from build123d import *

# Parameters (mm, degrees)
F0_R     = 1.35
F0_W     = 33.5
F0_H     = 25
F1_DEPTH = 15
F0_R_2   = 0.75
F0_W_2   = 24.5
F0_H_2   = 24.5
F2_DEPTH = 3
F3_DEPTH = 8
F4_DEPTH = 4


with BuildPart() as f1:
    # F0 (on Top) → F1 (new body)
    with BuildSketch(Plane.XY):
        with BuildLine():
            ThreePointArc((-20.740295, 15.731344), (-23.568722, 14.559771), (-24.740295, 11.731344))
            Line((-24.740295, 11.731344), (-24.740295, -20.268656))
            ThreePointArc((-24.740295, -20.268656), (-23.568722, -23.097083), (-20.740295, -24.268656))
            Line((-20.740295, -24.268656), (16.259705, -24.268656))
            ThreePointArc((16.259705, -24.268656), (19.088132, -23.097083), (20.259705, -20.268656))
            Line((20.259705, -20.268656), (20.259705, 11.731344))
            ThreePointArc((20.259705, 11.731344), (19.088132, 14.559771), (16.259705, 15.731344))
            Line((16.259705, 15.731344), (-20.740295, 15.731344))
        make_face()
        with Locations((-20.740295, -20.268656)):
            Circle(F0_R, mode=Mode.SUBTRACT)
        with Locations((16.259705, -20.268656)):
            Circle(F0_R, mode=Mode.SUBTRACT)
        with Locations((-20.740295, 11.731344)):
            Circle(F0_R, mode=Mode.SUBTRACT)
        with Locations((-2.240295, -4.268656)):
            Rectangle(F0_W, F0_H, mode=Mode.SUBTRACT)
        with Locations((16.259705, 11.731344)):
            Circle(F0_R, mode=Mode.SUBTRACT)
    extrude(amount=F1_DEPTH)

    # F0 (on Top) → F2 (join)
    with BuildSketch(Plane.XY):
        with Locations((-2.240295, -4.268656)):
            Rectangle(F0_W, F0_H)
        with Locations((-16.674155, -4.268656)):
            Circle(F0_R_2, mode=Mode.SUBTRACT)
        with Locations((-2.240295, -4.268656)):
            Rectangle(F0_W_2, F0_H_2, mode=Mode.SUBTRACT)
        with Locations((12.193565, -4.268656)):
            Circle(F0_R_2, mode=Mode.SUBTRACT)
    extrude(amount=F2_DEPTH)

    # F0 (on Top) → F3 (join)
    with BuildSketch(Plane.XY):
        with Locations((-16.674155, -4.268656)):
            Circle(F0_R_2)
        with Locations((12.193565, -4.268656)):
            Circle(F0_R_2)
    extrude(amount=F3_DEPTH)

    # F0 (on Top) → F4 (join)
    with BuildSketch(Plane.XY):
        with Locations((-20.740295, 11.731344)):
            Circle(F0_R)
        with Locations((16.259705, 11.731344)):
            Circle(F0_R)
        with Locations((16.259705, -20.268656)):
            Circle(F0_R)
        with Locations((-20.740295, -20.268656)):
            Circle(F0_R)
    extrude(amount=F4_DEPTH)


solid = f1.part
For this review, take the finished solid that the model builds, in its own axes (mm). A direction names the side the tool comes from. Round coordinates to 2 decimals unless told otherwise and drop trailing zeros. Loops run counter-clockwise (first coordinate to the right, second up) from the corner with the lowest first, then second, coordinate; pieces in that order, holes last. Notation, with made-up numbers: (67, 52) - (125, 52) arc R26 cw to (125, 85) - close; hole circle Ø11 at (-9.75, -26). An arc over 180 degrees is marked (long way). One line per question, with ' | ' between items.
Q1. Take a section at A-A (x = -12). Give the boundary of the cut face in (y, z), and give its area (4 significant figures).
Taken from the geometry:
outline: (-24.27, 0) - (-16.52, 0) - (-16.52, 3) - (-16.77, 3) - (-16.77, 15) - (-24.27, 15) - close; (7.98, 0) - (15.73, 0) - (15.73, 15) - (8.23, 15) - (8.23, 3) - (7.98, 3) - close | area: 226.5 mm²
Q2. Take a section at B-B (z = 11). Give the boundary of the cut face in (x, y).
Taken from the geometry:
outline: (-24.74, -20.27) arc R4 ccw to (-20.74, -24.27) - (16.26, -24.27) arc R4 ccw to (20.26, -20.27) - (20.26, 11.73) arc R4 ccw to (16.26, 15.73) - (-20.74, 15.73) arc R4 ccw to (-24.74, 11.73) - close; hole circle Ø2.7 at (-20.74, -20.27); hole circle Ø2.7 at (-20.74, 11.73); hole (-18.99, -16.77) - (14.51, -16.77) - (14.51, 8.23) - (-18.99, 8.23) - close; hole circle Ø2.7 at (16.26, -20.27); hole circle Ø2.7 at (16.26, 11.73)
Q3. For line 1 along X through (y, z) = (-10.5, 1.5); line 2 along X through (y, z) = (-5, 13.5); line 3 along Y through (x, z) = (-3.5, 6), list the stretches that pass through material, from the lowest coordinate up. Write a range as [from, to].
Taken from the geometry:
line 1: x = [-24.74, -14.49], [10.01, 20.26] | line 2: x = [-24.74, -18.99], [14.51, 20.26] | line 3: y = [-24.27, -16.77], [8.23, 15.73]
Q4. For pin 1 (1.5 mm diameter, centred on x = -18, y = 10, fed in from -Z); pin 2 (0.8 mm diameter, centred on x = 16, y = 12, fed in from +Z), all flat-tipped, find the tip position at first contact; note any pin that passes through.
Taken from the geometry:
pin 1: stops at z = 0 | pin 2: stops at z = 4
Q5. Take a section at D-D (z = 5). Give the boundary of the cut face in (x, y).
Taken from the geometry:
outline: (-24.74, -20.27) arc R4 ccw to (-20.74, -24.27) - (16.26, -24.27) arc R4 ccw to (20.26, -20.27) - (20.26, 11.73) arc R4 ccw to (16.26, 15.73) - (-20.74, 15.73) arc R4 ccw to (-24.74, 11.73) - close; circle Ø1.5 at (-16.67, -4.27); circle Ø1.5 at (12.19, -4.27); hole circle Ø2.7 at (-20.74, -20.27); hole circle Ø2.7 at (-20.74, 11.73); hole (-18.99, -16.77) - (14.51, -16.77) - (14.51, 8.23) - (-18.99, 8.23) - close; hole circle Ø2.7 at (16.26, -20.27); hole circle Ø2.7 at (16.26, 11.73)
Q6. Tool access review of faces 1 (the flat face through (-2, 7.981, 1)), 2 (the cylindrical face through (-23.54, 14.59, 7.4)), 3 (the flat face through (-18.99, -4, 9)): name each direction out of +Z, -Z, +X, -X, +Y, -Y from which nothing blocks a thin tool from reaching the whole face with its end or side.
Taken from the geometry:
face 1: +Z, -Z | face 2: +Z, -Z, -X, +Y | face 3: +Z
Q7. The part is to be moulded in two halves that separate along Y. For faces 4 (the flat face through (-15, -4, 3)), 5 (the cylindrical face through (19.12, 14.53, 7.4)), 6 (the flat face through (-3, 9, 15)), say which applies: released by +Y, released by -Y, zero draft, split by the parting line, or undercut.
Taken from the geometry:
face 4: undercut | face 5: released by +Y | face 6: zero draft
Q8. Take a section at C-C (y = -14.5). Give the boundary of the cut face in (x, z), and give its area (4 significant figures).
Taken from the geometry:
outline: (-24.74, 0) - (-14.49, 0) - (-14.49, 3) - (-18.99, 3) - (-18.99, 15) - (-24.74, 15) - close; (10.01, 0) - (20.26, 0) - (20.26, 15) - (14.51, 15) - (14.51, 3) - (10.01, 3) - close | area: 199.5 mm²
